Part print with two shaded views. Sizes in mm from the minimum x, y, z corner. Round coordinates to 2 decimals unless told otherwise and drop trailing zeros. Write each loop counter-clockwise with the first axis right and the second up, starting at its lowest first coordinate (ties: lowest second). Pieces come first, ordered by that corner, then holes. Notation, with made-up numbers: (18, -39) - (56, -39) arc R19 ccw to (56, -25) - close; hole circle Ø9 at (1.5, -37.5). An arc over 180 degrees is marked (long way). Use one line per item in the form item = value. Start each with the question number.
Item 1: Band-saw the part on C-C, the plane z = 1. List the corners of the cut face in (x, y), and give its area (3 significant figures).
Item 2: Drill centre lines: L1, parallel to Y at x = 15.25, z = 0.55; L2, parallel to Y at x = 11.5, z = 0.35; L3, parallel to X at y = 5.75, z = 0.8. Where is each one in solid material? Low to high.
Item 3: Band-saw the part on A-A, the plane y = 15. List the corners of the cut face in (x, z), and give its area (4 significant figures).
Item 4: Band-saw the part on D-D, the plane y = 6. List the corners of the cut face in (x, z).
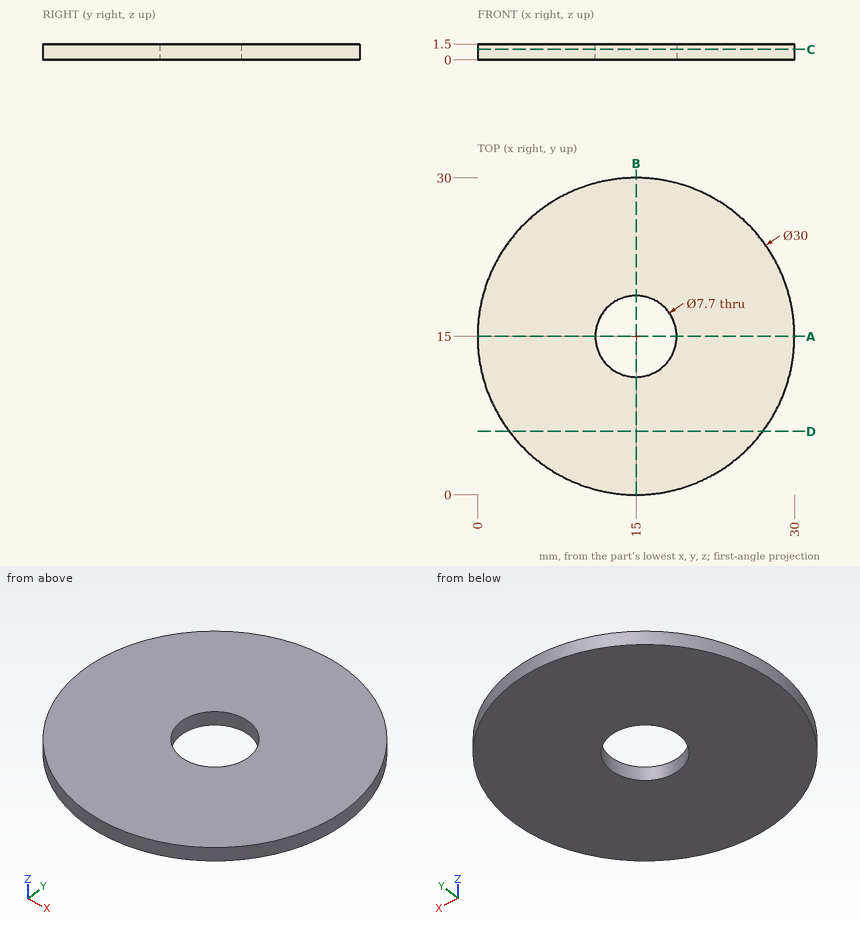
Determined:
q1.outline = circle Ø30 at (15, 15); hole circle Ø7.7 at (15, 15)
q1.area = 660 mm²
q2.L1 = 0 to 11.16, 18.84 to 30
q2.L2 = 0.41 to 13.4, 16.6 to 29.59
q2.L3 = 3.19 to 26.81
q3.outline = (0, 0) - (11.15, 0) - (11.15, 1.5) - (0, 1.5) - close; (18.85, 0) - (30, 0) - (30, 1.5) - (18.85, 1.5) - close
q3.area = 33.45 mm²
q4.outline = (3, 0) - (27, 0) - (27, 1.5) - (3, 1.5) - close
